from build123d import *

# Parameters (mm, degrees)
SKETCH1_W           = 37
SKETCH1_H           = 67
SKETCH1_R           = 1.5
BOSS_EXTRUDE1_DEPTH = 3
SKETCH2_W           = 6
SKETCH2_H           = 6
SKETCH2_R           = 1.5
BOSS_EXTRUDE2_DEPTH = 5
FILLET1_R           = 2
SKETCH3_W           = 20
SKETCH3_H           = 6
SKETCH3_R           = 1.5
BOSS_EXTRUDE3_DEPTH = 3
FILLET2_R           = 2
CHAMFER1_SIZE       = 1.55


with BuildPart() as part:
    # Sketch1 → Boss-Extrude1 (new body)
    with BuildSketch(Plane(origin=(0, 0, 0), x_dir=(1, 0, 0), z_dir=(0, 1, 0))):
        with Locations((-18, 33)):
            Rectangle(SKETCH1_W, SKETCH1_H)
        with Locations(Location((-2.5, 63.5, 0), (0, 0, 270))):
            Circle(SKETCH1_R, mode=Mode.SUBTRACT)
        with Locations(Location((-33.5, 63.5, 0), (0, 0, 270))):
            Circle(SKETCH1_R, mode=Mode.SUBTRACT)
        with Locations(Location((-2.5, 2.5, 0), (0, 0, 270))):
            Circle(SKETCH1_R, mode=Mode.SUBTRACT)
        with Locations(Location((-33.5, 2.5, 0), (0, 0, 270))):
            Circle(SKETCH1_R, mode=Mode.SUBTRACT)
    extrude(amount=BOSS_EXTRUDE1_DEPTH)

    # Sketch2 → Boss-Extrude2 (add)
    # profile 1 of 4: a face of its own
    with BuildSketch(Plane(origin=(0, 3, 0), x_dir=(1, 0, 0), z_dir=(0, 1, 0))):
        with Locations((-33.5, 63.5)):
            Rectangle(SKETCH2_W, SKETCH2_H)
        with Locations(Location((-33.5, 63.5, 0), (0, 0, 270))):
            Circle(SKETCH2_R, mode=Mode.SUBTRACT)
    # profile 2 of 4: a face of its own
    with BuildSketch(Plane(origin=(0, 3, 0), x_dir=(1, 0, 0), z_dir=(0, 1, 0))):
        with Locations((-2.5, 63.5)):
            Rectangle(SKETCH2_W, SKETCH2_H)
        with Locations(Location((-2.5, 63.5, 0), (0, 0, 270))):
            Circle(SKETCH2_R, mode=Mode.SUBTRACT)
    # profile 3 of 4: a face of its own
    with BuildSketch(Plane(origin=(0, 3, 0), x_dir=(1, 0, 0), z_dir=(0, 1, 0))):
        with Locations((-2.5, 2.5)):
            Rectangle(SKETCH2_W, SKETCH2_H)
        with Locations(Location((-2.5, 2.5, 0), (0, 0, 270))):
            Circle(SKETCH2_R, mode=Mode.SUBTRACT)
    # profile 4 of 4: a face of its own
    with BuildSketch(Plane(origin=(0, 3, 0), x_dir=(1, 0, 0), z_dir=(0, 1, 0))):
        with Locations((-33.5, 2.5)):
            Rectangle(SKETCH2_W, SKETCH2_H)
        with Locations(Location((-33.5, 2.5, 0), (0, 0, 270))):
            Circle(SKETCH2_R, mode=Mode.SUBTRACT)
    extrude(amount=BOSS_EXTRUDE2_DEPTH)

    # Fillet1
    fillet1_edges = [part.edges().sort_by_distance(p)[0] for p in [
        (0.5, 4, 0.5),
        (-36.5, 4, 0.5),
        (-36.5, 4, -66.5),
        (0.5, 4, -66.5),
        (-36.5, 5.5, -60.5),
        (-30.5, 5.5, -60.5),
        (-30.5, 5.5, -66.5),
        (0.5, 5.5, -60.5),
        (-5.5, 5.5, -66.5),
        (-5.5, 5.5, -60.5),
        (0.5, 5.5, -5.5),
        (-5.5, 5.5, -5.5),
        (-36.5, 5.5, -5.5),
        (-30.5, 5.5, -5.5),
    ]]
    fillet(fillet1_edges, radius=FILLET1_R)

    # Sketch3 → Boss-Extrude3 (add)
    # profile 1 of 2: a face of its own
    with BuildSketch(Plane(origin=(0, 3, 0), x_dir=(1, 0, 0), z_dir=(0, 1, 0))):
        with Locations((-18, 69.5)):
            Rectangle(SKETCH3_W, SKETCH3_H)
        with Locations(Location((-13, 69.5, 0), (0, 0, 270))):
            Circle(SKETCH3_R, mode=Mode.SUBTRACT)
        with Locations(Location((-23, 69.5, 0), (0, 0, 270))):
            Circle(SKETCH3_R, mode=Mode.SUBTRACT)
    # profile 2 of 2: a face of its own
    with BuildSketch(Plane(origin=(0, 3, 0), x_dir=(1, 0, 0), z_dir=(0, 1, 0))):
        with Locations((-18, -3.5)):
            Rectangle(SKETCH3_W, SKETCH3_H)
        with Locations(Location((-23, -3.5, 0), (0, 0, 270))):
            Circle(SKETCH3_R, mode=Mode.SUBTRACT)
        with Locations(Location((-13, -3.5, 0), (0, 0, 270))):
            Circle(SKETCH3_R, mode=Mode.SUBTRACT)
    extrude(amount=-BOSS_EXTRUDE3_DEPTH)

    # Fillet2
    fillet2_edges = [part.edges().sort_by_distance(p)[0] for p in [
        (-28, 1.5, 0.5),
        (-8, 1.5, 0.5),
        (-8, 1.5, 6.5),
        (-28, 1.5, 6.5),
        (-28, 1.5, -66.5),
        (-8, 1.5, -66.5),
        (-8, 1.5, -72.5),
        (-28, 1.5, -72.5),
    ]]
    fillet(fillet2_edges, radius=FILLET2_R)

    # Chamfer1
    # the kernel refuses this chamfer: 1.55 mm, written as the material it takes off along each edge
    with BuildSketch(Plane(origin=(-23, 3, 3.5), x_dir=(0, 0, 1), z_dir=(-1, 0, 0))) as chamfer1_piece_1:
        Polygon((1.5 + CHAMFER1_SIZE, 0), (1.5, -CHAMFER1_SIZE), (1.5, 0), align=None)
    revolve(axis=Axis((-23, 3, 3.5), (0, 1, 0)), mode=Mode.SUBTRACT)
    with BuildSketch(Plane(origin=(-13, 3, 3.5), x_dir=(0, 0, 1), z_dir=(-1, 0, 0))) as chamfer1_piece_2:
        Polygon((1.5 + CHAMFER1_SIZE, 0), (1.5, -CHAMFER1_SIZE), (1.5, 0), align=None)
    revolve(axis=Axis((-13, 3, 3.5), (0, 1, 0)), mode=Mode.SUBTRACT)
    with BuildSketch(Plane(origin=(-23, 3, -69.5), x_dir=(0, 0, 1), z_dir=(-1, 0, 0))) as chamfer1_piece_3:
        Polygon((1.5 + CHAMFER1_SIZE, 0), (1.5, -CHAMFER1_SIZE), (1.5, 0), align=None)
    revolve(axis=Axis((-23, 3, -69.5), (0, 1, 0)), mode=Mode.SUBTRACT)
    with BuildSketch(Plane(origin=(-13, 3, -69.5), x_dir=(0, 0, 1), z_dir=(-1, 0, 0))) as chamfer1_piece_4:
        Polygon((1.5 + CHAMFER1_SIZE, 0), (1.5, -CHAMFER1_SIZE), (1.5, 0), align=None)
    revolve(axis=Axis((-13, 3, -69.5), (0, 1, 0)), mode=Mode.SUBTRACT)


solid = part.part
The listing builds one solid part. Answer for the finished solid, in the listing's coordinates (mm). A direction names the side the tool comes from. Give positions to 0.01 mm unless a question says otherwise; leave off trailing zeros. Loops run counter-clockwise (first coordinate to the right, second up) from the corner with the lowest first, then second, coordinate; pieces in that order, holes last. Notation, with made-up numbers: (54.25, 61) - (84.25, 61) arc R26 cw to (84.25, 100) - close; hole circle Ø4 at (21.25, 34.25). An arc over 180 degrees is marked (long way). Write each question's results on one line, items separated by ' | '.
1. Find section B-B, the plane z = -2.5. Write down the section's boundary in (x, y).
Resolved:
outline: (-36.5, 0) - (-35, 0) - (-35, 8) - (-36.5, 8) - close; (-32, 0) - (-4, 0) - (-4, 8) - (-5.5, 8) - (-5.5, 3) - (-30.5, 3) - (-30.5, 8) - (-32, 8) - close; (-1, 0) - (0.5, 0) - (0.5, 8) - (-1, 8) - close
2. Flat-ended cylindrical pins translate along their axes: P1, Ø2.5, axis at x = -13, z = 3.5, coming from the +Y side; P2, Ø1, axis at x = -2.5, y = 6, coming from the -Z side; P3, Ø2, axis at y = 2, z = -70, coming from the -X side; P4, Ø18.5, axis at x = -26.5, z = -37.5, coming from the +Y side. Find the tip coordinate at first contact, or state that the pin passes through.
Resolved:
P1: passes through | P2: stops at z = -66.5 | P3: stops at x = -28 | P4: stops at y = 3
3. Find section A-A, the plane y = 6. Count the separate pieces of the cut face and the enclosed holes in it, then the cut area to 3 significant figures.
Resolved:
separate pieces: 4 | enclosed holes: 4 | area: 104 mm^2
4. Find section D-D, the plane z = -13.5. Write down the section's boundary in (x, y), then the cut area to 3 significant figures.
Resolved:
outline: (-36.5, 0) - (0.5, 0) - (0.5, 3) - (-36.5, 3) - close | area: 111 mm^2
5. Find section C-C, the plane x = -2.5. Write down the section's boundary in (y, z).
Resolved:
outline: (0, -66.5) - (8, -66.5) - (8, -65) - (0, -65) - close; (0, -62) - (8, -62) - (8, -60.5) - (3, -60.5) - (3, -5.5) - (8, -5.5) - (8, -4) - (0, -4) - close; (0, -1) - (8, -1) - (8, 0.5) - (0, 0.5) - close
6. Which of the six approach directions +Z, -Z, +X, -X, +Y, -Y give full straight-line access (tool end or side, diameter ignored) to faces 1 (the face through (-8, 2, 4)), 2 (the face through (-8, 2, -69)), 3 (the face through (-34, 5, -60.5)), 4 (the face through (-30.5, 5, -63)), 5 (the face through (-4.9, 5.54, -61.07))?
Resolved:
face 1: +Z, +X, +Y, -Y | face 2: -Z, +X, +Y, -Y | face 3: +X, -X, +Y | face 4: +Z, -Z, +Y | face 5: +Y
7. Consider probe 1 along X at (y, z) = (1.5, -63.5); probe 2 along X at (y, z) = (0.6, 3.5); probe 3 along X at (y, z) = (4, -2.5). Determine where each line is inside the solid, lowest interval first. Write a range as from..to.
Resolved:
probe 1: x = -36.5..-35, -32..-4, -1..0.5 | probe 2: x = -28..-24.5, -21.5..-14.5, -11.5..-8 | probe 3: x = -36.5..-35, -32..-30.5, -5.5..-4, -1..0.5
